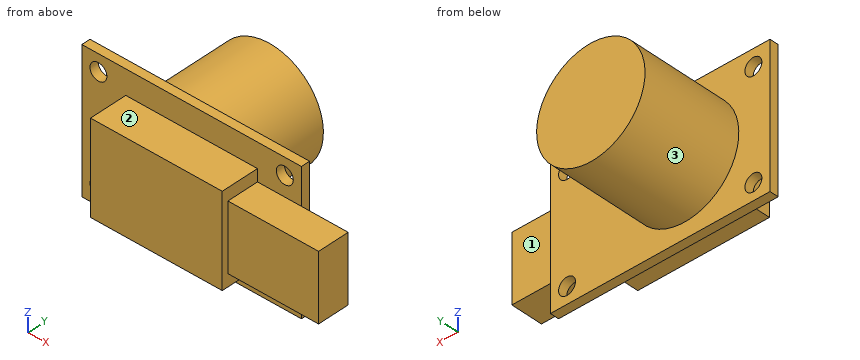
from build123d import *

# Parameters (mm, degrees)
SKETCH1_W           = 32.4
SKETCH1_H           = 20.55
SKETCH1_R           = 1.25
BOSS_EXTRUDE1_DEPTH = 1.3
SKETCH2_R           = 8
BOSS_EXTRUDE2_DEPTH = 14.9
SKETCH3_W           = 19.437089118
SKETCH3_H           = 13.404889048
BOSS_EXTRUDE3_DEPTH = 5.6
SKETCH4_W           = 13.8
SKETCH4_H           = 9.8
BOSS_EXTRUDE4_DEPTH = 4.7


with BuildPart() as part:
    # Sketch1 → Boss-Extrude1 (new body)
    with BuildSketch(Plane(origin=(0, 0, 0), x_dir=(1, 0, 0), z_dir=(0, 1, 0))):
        Rectangle(SKETCH1_W, SKETCH1_H)
        with Locations(Location((-13.75, 7.825, 0), (0, 0, 270))):
            Circle(SKETCH1_R, mode=Mode.SUBTRACT)
        with Locations(Location((-13.75, -7.825, 0), (0, 0, 90))):
            Circle(SKETCH1_R, mode=Mode.SUBTRACT)
        with Locations(Location((13.75, -7.825, 0), (0, 0, 270))):
            Circle(SKETCH1_R, mode=Mode.SUBTRACT)
        with Locations(Location((13.75, 7.825, 0), (0, 0, 90))):
            Circle(SKETCH1_R, mode=Mode.SUBTRACT)
    extrude(amount=BOSS_EXTRUDE1_DEPTH)

    # Sketch2 → Boss-Extrude2 (add)
    with BuildSketch(Plane(origin=(0, 1.3, 0), x_dir=(1, 0, 0), z_dir=(0, 1, 0))):
        with Locations(Location((-3.6, 0, 0), (0, 0, 270))):
            Circle(SKETCH2_R)
    extrude(amount=BOSS_EXTRUDE2_DEPTH)

    # Sketch3 → Boss-Extrude3 (add)
    with BuildSketch(Plane.XZ):
        Rectangle(SKETCH3_W, SKETCH3_H)
    extrude(amount=BOSS_EXTRUDE3_DEPTH)

    # Sketch4 → Boss-Extrude4 (add)
    with BuildSketch(Plane.XZ):
        with Locations((16.2, 0)):
            Rectangle(SKETCH4_W, SKETCH4_H)
    extrude(amount=BOSS_EXTRUDE4_DEPTH)


solid = part.part
Part model, mm, in its own coordinate system. Face numbers are marked on the shaded views. A direction names the side the tool comes from. Give positions to 0.01 mm unless a question says otherwise; leave off trailing zeros. Order: outer loops, then holes, each group sorted by start corner. A loop starts at its lowest first (then second) coordinate and runs counter-clockwise, first axis right, second up. Notation, with made-up numbers: (-7.75, 56) - (28.25, 56) arc R17 cw to (28.25, 71) - close; hole circle Ø10 at (15.25, -17). An arc over 180 degrees is marked (long way). One line per question, with ' | ' between items.
1. Band-saw the part on B-B on z = 0. List the corners of the cut face in (x, y).
Filled in:
outline: (-16.2, 0) - (-9.72, 0) - (-9.72, -5.6) - (9.72, -5.6) - (9.72, -4.7) - (23.1, -4.7) - (23.1, 0) - (16.2, 0) - (16.2, 1.3) - (4.4, 1.3) - (4.4, 16.2) - (-11.6, 16.2) - (-11.6, 1.3) - (-16.2, 1.3) - close
2. Band-saw the part on A-A on x = -13.75. List the corners of the cut face in (y, z) (3 decimals).
Filled in:
outline: (0, -10.275) - (1.3, -10.275) - (1.3, -9.075) - (0, -9.075) - close; (0, -6.575) - (1.3, -6.575) - (1.3, 6.575) - (0, 6.575) - close; (0, 9.075) - (1.3, 9.075) - (1.3, 10.275) - (0, 10.275) - close
3. Band-saw the part on C-C on y = -3.5. List the corners of the cut face in (x, z).
Filled in:
outline: (-9.72, -6.7) - (9.72, -6.7) - (9.72, -4.9) - (23.1, -4.9) - (23.1, 4.9) - (9.72, 4.9) - (9.72, 6.7) - (-9.72, 6.7) - close
4. Drop flat-ended pins along their axis: P1, Ø3, axis at x = -13.75, z = -7.825, coming from the -Y side; P2, Ø3, axis at x = -0.5, y = -2.5, coming from the -Z side; P3, Ø3, axis at y = 7.5, z = -6, coming from the +X side. Give the stop position or say it passes through.
Filled in:
P1: y = 0 | P2: z = -6.7 | P3: x = 3.01
5. Which spindle directions (+Z, -Z, +X, -X, +Y, -Y) get a long thin tool onto all of the face, cutting with end or side? Do the marked faces 1, 2 and 3. Say none if no direction does.
Filled in:
face 1: +Z, -Z, +X, +Y | face 2: +Z, +X, -X, -Y | face 3: +Y
6. Band-saw the part on D-D on x = 13.75. List the corners of the cut face in (y, z) (3 decimals).
Filled in:
outline: (-4.7, -4.9) - (0, -4.9) - (0, -6.575) - (1.3, -6.575) - (1.3, 6.575) - (0, 6.575) - (0, 4.9) - (-4.7, 4.9) - close; (0, -10.275) - (1.3, -10.275) - (1.3, -9.075) - (0, -9.075) - close; (0, 9.075) - (1.3, 9.075) - (1.3, 10.275) - (0, 10.275) - close
7. Drill centre lines: probe 1 along X at (y, z) = (-2.5, -4.25); probe 2 along Y at (x, z) = (14, -2.5); probe 3 along Z at (x, y) = (-0.5, -0.5). Where is each one in solid material? Low to high.
Filled in:
probe 1: -9.72 to 23.1 | probe 2: -4.7 to 1.3 | probe 3: -6.7 to 6.7
